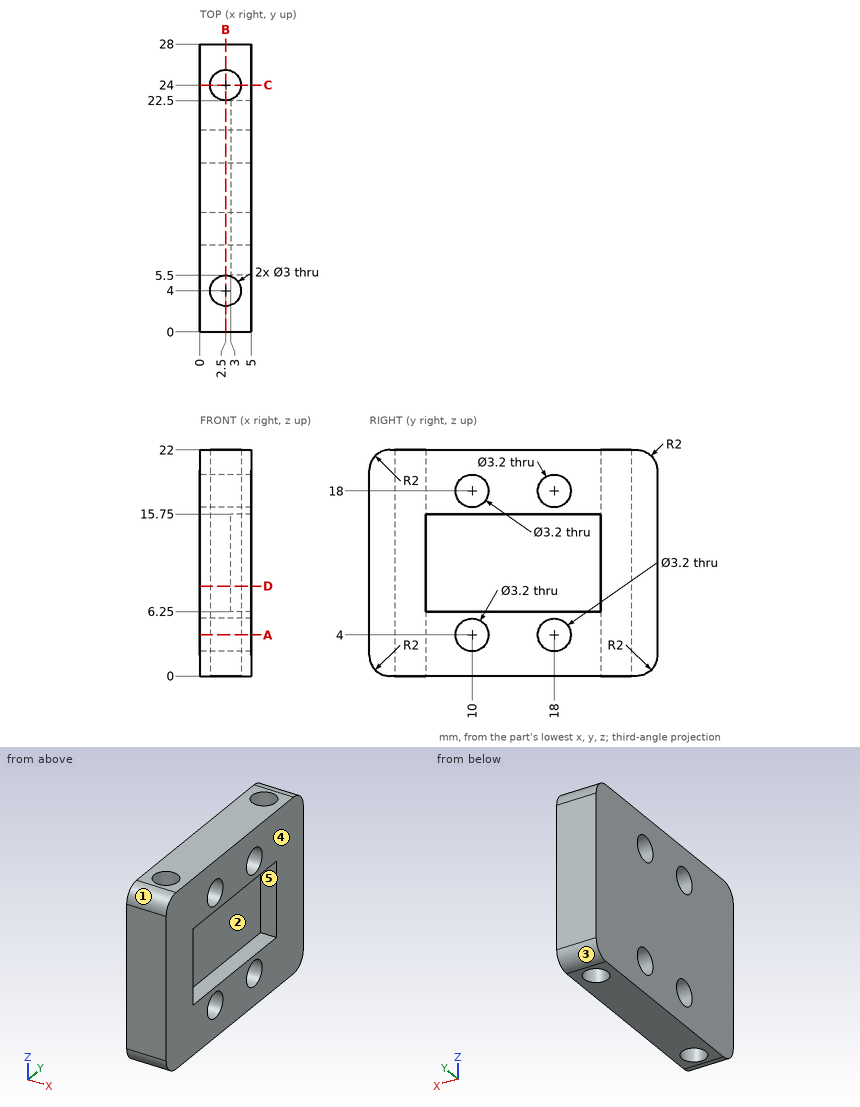
Could you check a few things on this drawing? It's one solid part, dimensions in mm from its lowest x, y, z. A direction names the side the tool comes from. Round coordinates to 2 decimals unless told otherwise and drop trailing zeros. Write each loop counter-clockwise with the first axis right and the second up, starting at its lowest first coordinate (ties: lowest second). Pieces come first, ordered by that corner, then holes. Notation, with made-up numbers: (63.25, -3) -> (113.25, -3) arc R22 ccw to (113.25, 10) -> close; hole circle Ø4 at (-8, -9.5). An arc over 180 degrees is marked (long way). Use a Markdown table: item, result.
1. If we section it at C-C (y = 24): List the corners of the cut face in (x, z) for me, then the cut area to 3 significant figures.
Answer key:
| item | result |
|---|---|
| outline | (0, 0) -> (1, 0) -> (1, 22) -> (0, 22) -> close; (4, 0) -> (5, 0) -> (5, 22) -> (4, 22) -> close |
| area | 44.0 mm^2 |
2. If we section it at A-A (z = 4): List the corners of the cut face in (x, y) for me.
Answer key:
| item | result |
|---|---|
| outline | (0, 0) -> (5, 0) -> (5, 8.4) -> (0, 8.4) -> close; (0, 11.6) -> (5, 11.6) -> (5, 16.4) -> (0, 16.4) -> close; (0, 19.6) -> (5, 19.6) -> (5, 28) -> (0, 28) -> close; hole circle Ø3 at (2.5, 4); hole circle Ø3 at (2.5, 24) |
3. Please list where these lines run through material, in increasing order: probe 1 along Y at (x, z) = (2.5, 12); probe 2 along Z at (x, y) = (2.6, 10); probe 3 along Z at (x, y) = (3.9, 18).
Answer key:
| item | result |
|---|---|
| probe 1 | y = 0 to 2.5, 5.5 to 22.5, 25.5 to 28 |
| probe 2 | z = 0 to 2.4, 5.6 to 16.4, 19.6 to 22 |
| probe 3 | z = 0 to 2.4, 5.6 to 6.25, 15.75 to 16.4, 19.6 to 22 |
4. Which directions (+Z, -Z, +X, -X, +Y, -Y) give clear straight access to the entire face, cutting with the end or side of a thin tool? Please do the marked faces 1 and 2.
Answer key:
| item | result |
|---|---|
| face 1 | +Z, +X, -X, -Y |
| face 2 | +X |
5. If we section it at D-D (z = 8.75): List the corners of the cut face in (x, y) for me.
Answer key:
| item | result |
|---|---|
| outline | (0, 0) -> (5, 0) -> (5, 5.5) -> (3, 5.5) -> (3, 22.5) -> (5, 22.5) -> (5, 28) -> (0, 28) -> close; hole circle Ø3 at (2.5, 4); hole circle Ø3 at (2.5, 24) |
6. If we section it at B-B (x = 2.5): List the corners of the cut face in (y, z) for me.
Answer key:
| item | result |
|---|---|
| outline | (0, 2) arc R2 ccw to (2, 0) -> (2.5, 0) -> (2.5, 22) -> (2, 22) arc R2 ccw to (0, 20) -> close; (5.5, 0) -> (22.5, 0) -> (22.5, 22) -> (5.5, 22) -> close; (25.5, 0) -> (26, 0) arc R2 ccw to (28, 2) -> (28, 20) arc R2 ccw to (26, 22) -> (25.5, 22) -> close; hole circle Ø3.2 at (10, 4); hole circle Ø3.2 at (10, 18); hole circle Ø3.2 at (18, 4); hole circle Ø3.2 at (18, 18) |
7. For pin 1 Ø3 at (y, z) = (18, 4) entering from +X, with a flat end and sliding along its axis, tell me the tip position at first contact or that it passes through.
Answer key:
| item | result |
|---|---|
| pin 1 | passes through |
8. We'd pull the mould along Y, two halves only. Please class the marked faces 3, 4 and 5: +Y half, -Y half, draft (parallel to the pull), parting line (faces both ways), or undercut.
Answer key:
| item | result |
|---|---|
| face 3 | +Y half |
| face 4 | draft |
| face 5 | undercut |
